Autodesk Inventor part; units mm, degrees
ref_plane "YZ Plane" through (0, 0, 0) normal (1, 0, 0) x (0, 1, 0)
ref_plane "XZ Plane" through (0, 0, 0) normal (0, 1, 0) x (-1, 0, 0)
ref_plane "XY Plane" through (0, 0, 0) normal (0, 0, 1) x (1, 0, 0)
sketch "Sketch1" plane through (0, 0, 0) normal (0, 0, 1) x (1, 0, 0)
  line L0 (-219.6419, 61.3316) -> (-117.215, 61.3316)
  line L1 (-117.215, 61.3316) -> (-117.215, -56.6617)
  line L2 (-117.215, -56.6617) -> (-219.6419, -56.6617)
  line L3 (-219.6419, -56.6617) -> (-219.6419, 61.3316)
  point P0 (0, 0)
extrude "Extrusion1" add sketch "Sketch1" along normal blind 10
sketch "Sketch2" plane through (0, 0, 10) normal (0, 0, 1) x (1, 0, 0)
  line L0 (-165.5966, 48.7171) -> (-165.5966, -16.2829) construction
  line L1 (-171.5966, 42.7171) -> (-171.5966, -10.2829)
  line L2 (-159.5966, -10.2829) -> (-159.5966, 42.7171)
  arc A0 (-159.5966, 42.7171) -> (-171.5966, 42.7171) centre (-165.5966, 42.7171) ccw
  arc A1 (-171.5966, -10.2829) -> (-159.5966, -10.2829) centre (-165.5966, -10.2829) ccw
  point P0 (0, 0)
  point P1 (-165.5966, 16.2171)
  dimension "d2" = 12
  dimension "d3" = 65
extrude "Extrusion2" cut sketch "Sketch2" against normal through all
properties part number "belt circufrence"
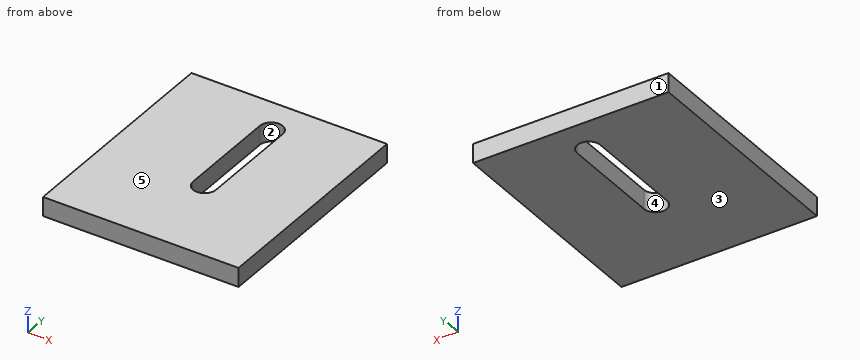
Read the model definition and answer for the solid it produces. Units are mm, in the model's axes. Face numbers are marked on the shaded views. A direction names the side the tool comes from. Round coordinates to 2 decimals unless told otherwise and drop trailing zeros. Write each loop counter-clockwise with the first axis right and the second up, starting at its lowest first coordinate (ties: lowest second). Pieces come first, ordered by that corner, then holes. Notation, with made-up numbers: (27.25, -35.75) - (39.25, -35.75) arc R21 cw to (39.25, 0.25) - close; hole circle Ø8 at (-2, 32.5). An arc over 180 degrees is marked (long way). One line per item, written item: value.
Q1. Find section B-B (z = 5.5). Determine the outline of the cut face in (x, y) (3 decimals).
The answers:
outline: (-219.642, -56.662) - (-117.215, -56.662) - (-117.215, 61.332) - (-219.642, 61.332) - close; hole (-171.597, -10.283) arc R6 ccw to (-159.597, -10.283) - (-159.597, 42.717) arc R6 ccw to (-171.597, 42.717) - close
Q2. Find section A-A (y = -0.5). Determine the outline of the cut face in (x, z) (3 decimals), and give its area (3 significant figures).
The answers:
outline: (-219.642, 0) - (-171.597, 0) - (-171.597, 10) - (-219.642, 10) - close; (-159.597, 0) - (-117.215, 0) - (-117.215, 10) - (-159.597, 10) - close
area: 904 mm2
Q3. Find section C-C (x = -167). Determine the outline of the cut face in (y, z).
The answers:
outline: (-56.66, 0) - (-16.12, 0) - (-16.12, 10) - (-56.66, 10) - close; (48.55, 0) - (61.33, 0) - (61.33, 10) - (48.55, 10) - close
Q4. For a pull along Y with two mould halves and no side action, classify the marked faces 1, 2 and 3 as pulls with the +Y half, pulls with the -Y half, needs draft (parallel to the pull), parting line crosses it, or undercut.
The answers:
face 1: pulls with the +Y half
face 2: undercut
face 3: needs draft
Q5. Straight lines are drawn through the part: line 1 (X direction, y = 39.5, z = 2) (3 decimals); line 2 (X direction, y = -15.5, z = 1) (3 decimals). For each, find the intervals that lie inside material, in ascending order. Write a range as from..to.
The answers:
line 1: x = -219.642..-171.597, -159.597..-117.215
line 2: x = -219.642..-168.56, -162.633..-117.215
Q6. Which of the six approach directions +Z, -Z, +X, -X, +Y, -Y give full straight-line access (tool end or side, diameter ignored) to the marked faces 4 and 5?
The answers:
face 4: +Z, -Z
face 5: +Z, +X, -X, +Y, -Y
